The listing builds one solid part. Answer for the finished solid, in the listing's coordinates (mm). Give positions to 0.01 mm unless a question says otherwise; leave off trailing zeros. Order: outer loops, then holes, each group sorted by start corner. A loop starts at its lowest first (then second) coordinate and runs counter-clockwise, first axis right, second up. Notation, with made-up numbers: (84, 50.5) - (135, 50.5) arc R29 cw to (135, 77.5) - close; hole circle Ø2 at (3, 56.25). An arc over 180 degrees is marked (long way). Use CSV: the item, a comma, the result in double quotes.
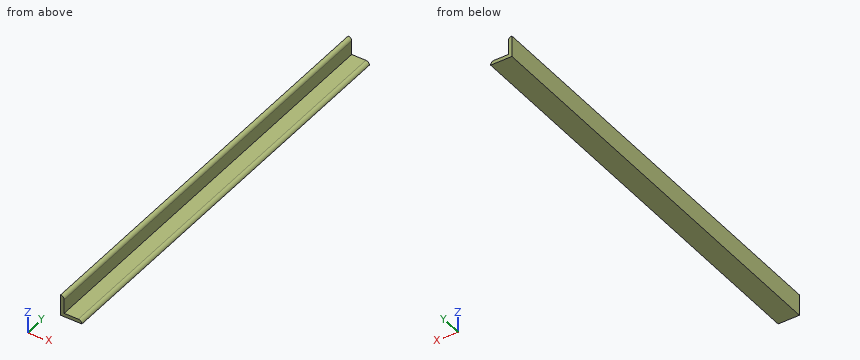
```python
from build123d import *

# Parameters (mm, degrees)
F1_DEPTH = 190.5


with BuildPart() as f1:
    # F0 (on Front) → F1 (new body, symmetric)
    with BuildSketch(Plane.XZ):
        with BuildLine():
            ThreePointArc((3.175, 15.875), (2.245064, 18.120064), (0, 19.05))
            Line((0, 19.05), (0, 0))
            Line((0, 0), (19.05, 0))
            ThreePointArc((19.05, 0), (18.120064, 2.245064), (15.875, 3.175))
            Line((15.875, 3.175), (3.175, 3.175))
            Line((3.175, 3.175), (3.175, 15.875))
        make_face()
    extrude(amount=F1_DEPTH, both=True)


solid = f1.part
```
Item 1: The part is cut by section A-A (z = 11.5). Give the vertices of the cut face in (x, y) (3 decimals), and give its area (3 significant figures).
Taken from the geometry:
outline,"(0, -190.5) - (3.175, -190.5) - (3.175, 190.5) - (0, 190.5) - close"
area,"1,210 mm^2"
Item 2: Each of these flat-tipped pins is pushed along its axis until it touches: pin 1 (6 mm diameter, centred on x = 16, y = 99.5, fed in from +Z) (3 decimals); pin 2 (1.5 mm diameter, centred on y = -104.5, z = 6.5, fed in from +X) (3 decimals). Where does it stop, or does it pass through?
Taken from the geometry:
pin 1,"z = 3.175"
pin 2,"x = 3.175"
Item 3: Find the intervals of material crossed by line 1 along Z through (x, y) = (11, 151) (3 decimals); line 2 along X through (y, z) = (123.5, 2.5), in increasing order.
Taken from the geometry:
line 1,"0 to 3.175"
line 2,"0 to 17.83"
Item 4: The part is cut by section B-B (y = -156.5). Give the vertices of the cut face in (x, z) (3 decimals), and give its area (3 significant figures).
Taken from the geometry:
outline,"(0, 0) - (19.05, 0) arc R3.175 ccw to (15.875, 3.175) - (3.175, 3.175) - (3.175, 15.875) arc R3.175 ccw to (0, 19.05) - close"
area,"107 mm^2"
Item 5: The part is cut by section C-C (x = 6.5). Give the vertices of the cut face in (y, z) (3 decimals), and give its area (3 significant figures).
Taken from the geometry:
outline,"(-190.5, 0) - (190.5, 0) - (190.5, 3.175) - (-190.5, 3.175) - close"
area,"1,210 mm^2"
